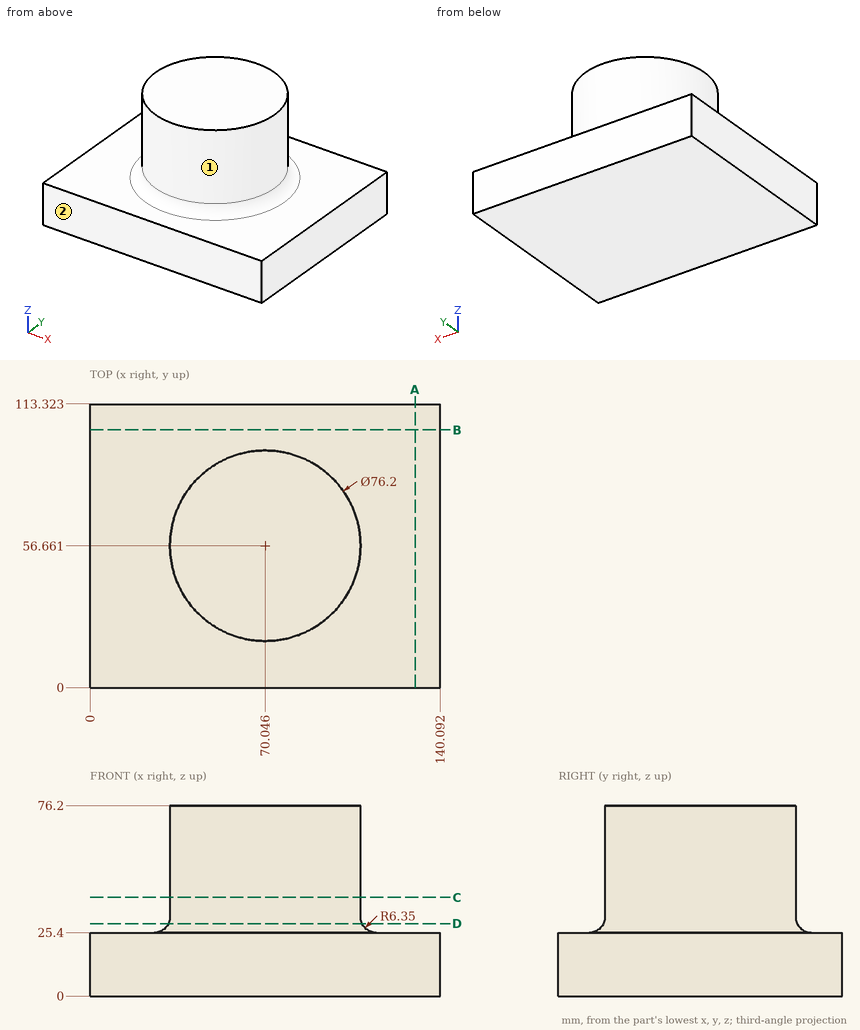
Input: dimensioned drawing with shaded views. Units: mm. Origin: part minimum x, y, z. A direction names the side the tool comes from. Coordinates: 2 decimals unless noted, no trailing zeros. Loops run counter-clockwise (first coordinate to the right, second up) from the corner with the lowest first, then second, coordinate; pieces in that order, holes last. Notation, with made-up numbers: M 14.25,-29 L 54.25,-29 A19 cw 54.25,-5 Z; hole C 22.5,61 d1. An arc over 180 degrees is marked long. Use a Markdown table: item, result. Add a question column.
Q1. Section query C-C, the plane z = 39.5. Return loops of the section in (x, y), and give its area (3 significant figures).
Q2. Material intervals for L1, parallel to Z at x = 7.5, y = 10.5; L2, parallel to Z at x = 90.5, y = 93; L3, parallel to Y at x = 85, z = 55 (1 decimal), sorted ascending.
Q3. Section query A-A, the plane x = 130. Return loops of the section in (y, z).
Q4. Section query B-B, the plane y = 103. Return loops of the section in (x, z), and give its area (3 significant figures).
Q5. Access query for the marked faces 1 and 2. Directions: +Z, -Z, +X, -X, +Y, -Y. A direction counts if a zero-diameter tool reaches every point of the face in a straight line with its end or side. Return the directions, or none.
Q6. First-contact query: pin 1 (10 mm diameter, centred on y = 87, z = 38.5, fed in from -X); pin 2 (3 mm diameter, centred on y = 85, z = 29, fed in from -X) (1 decimal); pin 3 (1 mm diameter, centred on x = 18, y = 20, fed in from +Z). Flat tips, straight axial feed; report the tip coordinate or a pass-through.
Q7. Section query D-D, the plane z = 29. Return loops of the section in (x, y), and give its area (3 significant figures).
Result:
| question | item | result |
|---|---|---|
| 1 | outline | C 70.05,56.66 d76.2 |
| 1 | area | 4,560 mm2 |
| 2 | L1 | z = 0 to 25.4 |
| 2 | L2 | z = 0 to 26.03 |
| 2 | L3 | y = 21.6 to 91.7 |
| 3 | outline | M 0,0 L 113.32,0 L 113.32,25.4 L 0,25.4 Z |
| 4 | outline | M 0,0 L 140.09,0 L 140.09,25.4 L 0,25.4 Z |
| 4 | area | 3,560 mm2 |
| 5 | face 1 | +Z |
| 5 | face 2 | +Z, -Z, +X, -X, -Y |
| 6 | pin 1 | stops at x = 41.59 |
| 6 | pin 2 | stops at x = 41.7 |
| 6 | pin 3 | stops at z = 25.4 |
| 7 | outline | C 70.05,56.66 d77.45 |
| 7 | area | 4,710 mm2 |
